from build123d import *

# Parameters (mm, degrees)
F1_DEPTH = 2.2098
F2_R     = 1.27
F4_DEPTH = 2.1844
F5_R     = 1.016


with BuildPart() as f1:
    # F0 (on Top) → F1 (new body)
    with BuildSketch(Plane.XY):
        with BuildLine():
            ThreePointArc((10.680274663, 22.1913547378), (11.3792147126, 24.4270132399), (11.6153963278, 26.7574433237))
            ThreePointArc((11.6153963278, 26.7574433237), (-2.3304300838, 38.1366580363), (-10.680274663, 22.1913547378))
            ThreePointArc((-10.680274663, 22.1913547378), (-9.0390071452, 19.4626656245), (-6.7184275333, 17.282203837))
            ThreePointArc((-6.7184275333, 17.282203837), (0, 22.1931135695), (6.7184275333, 17.282203837))
            ThreePointArc((6.7184275333, 17.282203837), (9.0390071452, 19.4626656245), (10.680274663, 22.1913547378))
        make_face()
        with BuildLine():
            ThreePointArc((6.7184275333, 17.282203837), (0, 22.1931135695), (-6.7184275333, 17.282203837))
            ThreePointArc((-6.7184275333, 17.282203837), (0, 15.142046996), (6.7184275333, 17.282203837))
        make_face()
        with BuildLine():
            ThreePointArc((6.7184275333, 17.282203837), (0, 15.142046996), (-6.7184275333, 17.282203837))
            ThreePointArc((-6.7184275333, 17.282203837), (-7.0463335637, 14.8837387803), (-6.5436952619, 12.5157202562))
            Line((-6.5436952619, 12.5157202562), (-6.4198818287, 12.2261153899))
            Line((-6.4198818287, 12.2261153899), (6.4198818287, 12.2261153899))
            Line((6.4198818287, 12.2261153899), (6.5436952619, 12.5157202562))
            ThreePointArc((6.5436952619, 12.5157202562), (6.9230618499, 13.8046037456), (7.0510665736, 15.142046996))
            ThreePointArc((7.0510665736, 15.142046996), (6.9674105531, 16.2249735904), (6.7184275333, 17.282203837))
        make_face()
        with BuildLine():
            ThreePointArc((-6.7184275333, 17.282203837), (-9.0390071452, 19.4626656245), (-10.680274663, 22.1913547378))
            Line((-10.680274663, 22.1913547378), (-6.5436952619, 12.5157202562))
            ThreePointArc((-6.5436952619, 12.5157202562), (-7.0463335637, 14.8837387803), (-6.7184275333, 17.282203837))
        make_face()
        with BuildLine():
            Line((6.4198818287, 12.2261153899), (-6.4198818287, 12.2261153899))
            ThreePointArc((-6.4198818287, 12.2261153899), (0, 8.0909804224), (6.4198818287, 12.2261153899))
        make_face()
        with BuildLine():
            Line((6.5436952619, 12.5157202562), (10.680274663, 22.1913547378))
            ThreePointArc((10.680274663, 22.1913547378), (9.0390071452, 19.4626656245), (6.7184275333, 17.282203837))
            ThreePointArc((6.7184275333, 17.282203837), (6.9674105531, 16.2249735904), (7.0510665736, 15.142046996))
            ThreePointArc((7.0510665736, 15.142046996), (6.9230618499, 13.8046037456), (6.5436952619, 12.5157202562))
        make_face()
    extrude(amount=F1_DEPTH)

    # F2
    f2_edges = [f1.edges().sort_by_distance(p)[0] for p in [
        (8.550078, 17.208735, 2.2098),
        (0, 38.37284, 2.2098),
        (-8.550078, 17.208735, 2.2098),
        (0, 8.09098, 2.2098),
    ]]
    fillet(f2_edges, radius=F2_R)

    # F3 (on face) → F4 (join)
    with BuildSketch(Plane.XY.offset(2.2098)):
        with BuildLine():
            Line((0, 26.7574433237), (0, 36.074007986))
            ThreePointArc((0, 36.074007986), (-6.5878060501, 33.3452493738), (-9.3165646623, 26.7574433237))
            Line((-9.3165646623, 26.7574433237), (0, 26.7574433237))
        make_face()
        with BuildLine():
            ThreePointArc((9.3165646623, 26.7574433237), (6.5878060501, 33.3452493738), (0, 36.074007986))
            Line((0, 36.074007986), (0, 26.7574433237))
            Line((0, 26.7574433237), (0, 17.4408786614))
            ThreePointArc((0, 17.4408786614), (6.5878060501, 20.1696372737), (9.3165646623, 26.7574433237))
        make_face()
    extrude(amount=F4_DEPTH)

    # F5
    f5_edges = [f1.edges().sort_by_distance(p)[0] for p in [
        (6.587806, 33.345249, 4.3942),
    ]]
    fillet(f5_edges, radius=F5_R)


solid = f1.part
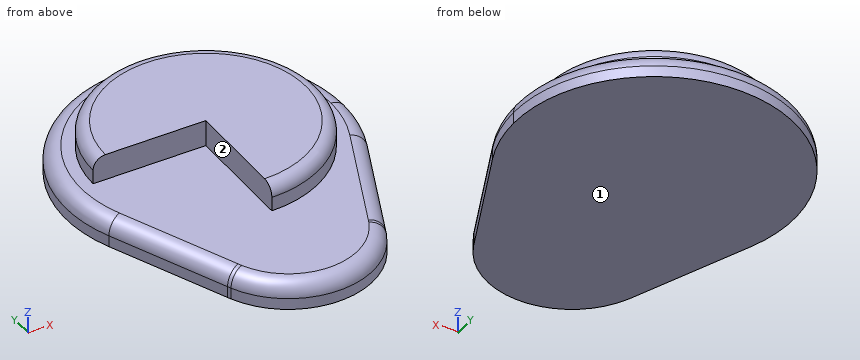
Design review of the part built by this model. Coordinates are the model's own, in mm. Face numbers are marked on the shaded views. A direction names the side the tool comes from. Round coordinates to 2 decimals unless told otherwise and drop trailing zeros. Write each loop counter-clockwise with the first axis right and the second up, starting at its lowest first coordinate (ties: lowest second). Pieces come first, ordered by that corner, then holes. Notation, with made-up numbers: (69.5, 22.25) - (101.5, 22.25) arc R21 cw to (101.5, 46.25) - close; hole circle Ø7 at (-34, -39). An arc over 180 degrees is marked (long way). Use a Markdown table: item, result. Add a question column.
1. We need section B-B (z = 3.95). State the section outline as (x, y) points, then the cut area to 3 significant figures.
2. Wall thickness on probe 1 along Z at (x, y) = (-0.5, 26); probe 2 along Y at (x, z) = (-4.75, 3.9); probe 3 along X at (y, z) = (31.5, 3.8): over which ranges is each line inside the solid? List them lowest first.
3. For the marked faces 1 and 2, list the 3-axis set-ups (+Z, -Z, +X, -X, +Y, -Y) from which the entire face can be reached by the end or side of a thin tool; tool diameter is ignored.
4. We need section A-A (z = 1.8). State the section outline as (x, y) points, then the cut area to 3 significant figures.
5. Clearance check with flat-ended pins moving along their axes: pin 1 (2 mm diameter, centred on y = 18.5, z = 4, fed in from +X); pin 2 (8 mm diameter, centred on x = -4, y = 34.5, fed in from +Z); pin 3 (1.1 mm diameter, centred on y = 20.5, z = 3.5, fed in from -X); pin 4 (5 mm diameter, centred on x = -5, y = 21, fed in from +Z). State where each tip first meets the part, or that it passes through.
Output:
| question | item | result |
|---|---|---|
| 1 | outline | (-9.14, 26.76) - (0, 26.76) - (0, 17.62) arc R9.14 ccw (long way) to start |
| 1 | area | 197 mm2 |
| 2 | probe 1 | z = 0 to 2.21 |
| 2 | probe 2 | y = 26.76 to 34.6 |
| 2 | probe 3 | x = -7.91 to 7.91 |
| 3 | face 1 | -Z, +X, -X, +Y, -Y |
| 3 | face 2 | +Z, -X, -Y |
| 4 | outline | (-10.37, 22.32) - (-6.11, 12.36) arc R6.72 ccw to (6.11, 12.36) - (10.37, 22.32) arc R11.28 ccw (long way) to start |
| 4 | area | 496 mm2 |
| 5 | pin 1 | stops at x = 5.7 |
| 5 | pin 2 | stops at z = 4.39 |
| 5 | pin 3 | stops at x = 0 |
| 5 | pin 4 | stops at z = 2.21 |
